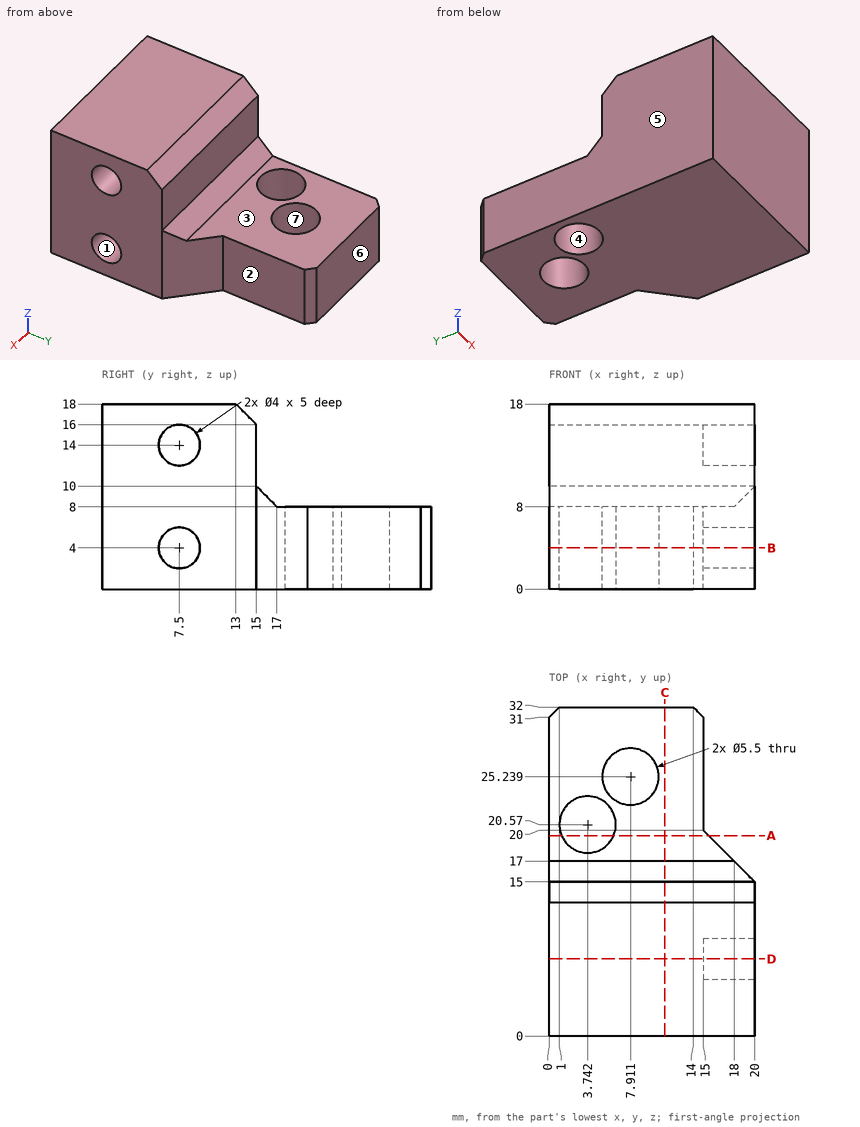
Check sheet for the drawn part. Datum: minimum x, y, z corner. Units: mm. A direction names the side the tool comes from. Coordinates: 2 decimals unless noted, no trailing zeros. Loops run counter-clockwise (first coordinate to the right, second up) from the corner with the lowest first, then second, coordinate; pieces in that order, holes last. Notation, with made-up numbers: (-10.75, -1) -> (42.25, -1) arc R8 ccw to (42.25, 13) -> close; hole circle Ø6 at (-18, 8.5). An arc over 180 degrees is marked (long way). Answer as a JSON object with one key per item and string values. Group by question number.
Item 1: Scan lines: probe 1 along Y at (x, z) = (12.75, 12.75); probe 2 along Z at (x, y) = (14.75, 28); probe 3 along X at (y, z) = (25.5, 1.5). Record each from-to range of solid material in increasing order.
Item 2: Sectioned sample at A-A on y = 19.5. Record the boundary of the cut face in (x, z) (1 decimal).
Item 3: Sectioned sample at B-B on z = 4. State how many separate pieces and enclosed holes the cut face has, plus the area to 3 significant figures.
Item 4: Sectioned sample at D-D on y = 7.5. Record the boundary of the cut face in (x, z), plus the area to 3 significant figures.
Item 5: Depth check by flat-ended pin: pin 1 (4.5 mm diameter, centred on x = 7.91, y = 25.24, fed in from +Z); pin 2 (7.5 mm diameter, centred on x = 9.5, y = 27, fed in from +Z); pin 3 (1.2 mm diameter, centred on y = 7, z = 3, fed in from +X); pin 4 (1.5 mm diameter, centred on x = 9, y = 17.5, fed in from +Z). Enter the tip coordinate at first touch or a pass-through.
Item 6: Mould release check, pull along Y, two halves, no side actions. Record for the marked faces 5, 6 and 7: +Y half, -Y half, draft (parallel to the pull), parting line (faces both ways), or undercut.
Item 7: Sectioned sample at C-C on x = 11.25. Record the boundary of the cut face in (y, z), plus the area to 3 significant figures.
Item 8: Tool access check on the marked faces 1, 2, 3 and 4. Record the directions out of +Z, -Z, +X, -X, +Y, -Y that give a thin tool (end or side, any length) a straight path to the whole face; none if there is none.
Evaluation:
{
 "1": {"probe 1": "y = 0 to 15", "probe 2": "z = 0 to 8", "probe 3": "x = 0 to 5.17, 10.65 to 15"},
 "2": {"outline": "(0, 0) -> (1.2, 0) -> (1.2, 8) -> (0, 8) -> close; (6.3, 0) -> (15.5, 0) -> (15.5, 8) -> (6.3, 8) -> close"},
 "3": {"separate pieces": "1", "enclosed holes": "2", "area": "499 mm²"},
 "4": {"outline": "(0, 0) -> (20, 0) -> (20, 2) -> (15, 2) -> (15, 6) -> (20, 6) -> (20, 12) -> (15, 12) -> (15, 16) -> (20, 16) -> (20, 18) -> (0, 18) -> close", "area": "320 mm²"},
 "5": {"pin 1": "passes through", "pin 2": "stops at z = 8", "pin 3": "stops at x = 15", "pin 4": "stops at z = 8.25"},
 "6": {"face 5": "draft", "face 6": "+Y half", "face 7": "undercut"},
 "7": {"outline": "(0, 0) -> (32, 0) -> (32, 8) -> (17, 8) -> (15, 10) -> (15, 16) -> (13, 18) -> (0, 18) -> close", "area": "406 mm²"},
 "8": {"face 1": "+X", "face 2": "+Z, -Z, +X, +Y", "face 3": "+Z, +X, -X, +Y", "face 4": "+Z, -Z"}
}
